from build123d import *

# Parameters (mm, degrees)
SKETCH1_W                                        = 55
SKETCH1_H                                        = 30
BOSS_EXTRUDE1_DEPTH                              = 10
SKETCH3_W                                        = 16.992180867
SKETCH3_H                                        = 11.731003527
SKETCH3_W_2                                      = 16.707792902
SKETCH3_W_3                                      = 9.029317866
SKETCH3_H_2                                      = 11.700356954
CUT_EXTRUDE1_DEPTH                               = 33.882366095
CBORE_FOR_M2_HEX_HEAD_MACHINE_SCREW2_D           = 2.4
CBORE_FOR_M2_HEX_HEAD_MACHINE_SCREW2_CBORE_D     = 6.38
CBORE_FOR_M2_HEX_HEAD_MACHINE_SCREW2_CBORE_DEPTH = 1.6
M3X0_5_TAPPED_HOLE3_D                            = 2.5
M3X0_5_TAPPED_HOLE3_DEPTH                        = 3
M3X0_5_TAPPED_HOLE3_TIP                          = 0.751075774


with BuildPart() as part:
    # Sketch1 → Boss-Extrude1 (new body)
    with BuildSketch(Plane.XY):
        Rectangle(SKETCH1_W, SKETCH1_H)
    extrude(amount=BOSS_EXTRUDE1_DEPTH)

    # Sketch3 → Cut-Extrude1 (cut, through all)
    with BuildSketch(Plane.XY.offset(10)):
        with Locations((-16.316759452, 0.350583033)):
            Rectangle(SKETCH3_W, SKETCH3_H)
        with Locations((4.016979996, 0.421680025)):
            Rectangle(SKETCH3_W_2, SKETCH3_H)
        with Locations((20.938063871, 0.193065764)):
            Rectangle(SKETCH3_W_3, SKETCH3_H_2)
    extrude(amount=-CUT_EXTRUDE1_DEPTH, mode=Mode.SUBTRACT)

    # CBORE for M2 Hex Head Machine Screw2 (through all)
    with Locations(Plane.XY.offset(10)):
        with Locations((-22.5, -10.5), (22.5, -10.5)):
            CounterBoreHole(CBORE_FOR_M2_HEX_HEAD_MACHINE_SCREW2_D / 2, CBORE_FOR_M2_HEX_HEAD_MACHINE_SCREW2_CBORE_D / 2, CBORE_FOR_M2_HEX_HEAD_MACHINE_SCREW2_CBORE_DEPTH)

    # M3x0.5 Tapped Hole3
    with Locations(Plane(origin=(0, 15, 0), x_dir=(1, 0, 0), z_dir=(0, 1, 0))):
        with Locations((-20.191545465, -5), (20.191545465, -5)):
            Hole(M3X0_5_TAPPED_HOLE3_D / 2, depth=M3X0_5_TAPPED_HOLE3_DEPTH)
            with Locations((0, 0, -(M3X0_5_TAPPED_HOLE3_DEPTH + M3X0_5_TAPPED_HOLE3_TIP / 2))):  # 118° drill point
                Cone(0, M3X0_5_TAPPED_HOLE3_D / 2, M3X0_5_TAPPED_HOLE3_TIP, mode=Mode.SUBTRACT)

    # Sketch12 → M3x0.5 Tapped Hole2 (revolve, cut)
    with BuildSketch(Plane(origin=(-27.5, -10, 5), x_dir=(0, 0, 1), z_dir=(0, 1, 0))):
        Polygon((0, 0), (0, 3.751075774), (1.25, 3), (1.25, 0), align=None)
    m3x0_5_tapped_hole2 = revolve(axis=Axis((-33.85, -10, 5), (1, 0, 0)), mode=Mode.SUBTRACT)

    # Sketch16 → M3x0.5 Tapped Hole1 (revolve, cut)
    with BuildSketch(Plane(origin=(27.5, -10, 5), x_dir=(0, 0, -1), z_dir=(0, 1, 0))):
        Polygon((0, 0), (0, 3.751075774), (1.25, 3), (1.25, 0), align=None)
    m3x0_5_tapped_hole1 = revolve(axis=Axis((33.85, -10, 5), (-1, 0, 0)), mode=Mode.SUBTRACT)

    # Mirror1: M3x0.5 Tapped Hole1 across plane
    add(m3x0_5_tapped_hole1.mirror(Plane.ZX), mode=Mode.SUBTRACT)

    # Mirror2: M3x0.5 Tapped Hole2 across plane
    add(m3x0_5_tapped_hole2.mirror(Plane.ZX), mode=Mode.SUBTRACT)


solid = part.part
Work out the finished part from the listing and answer in its coordinate system (mm). A direction names the side the tool comes from. Give positions to 0.01 mm unless a question says otherwise; leave off trailing zeros. Loops run counter-clockwise (first coordinate to the right, second up) from the corner with the lowest first, then second, coordinate; pieces in that order, holes last. Notation, with made-up numbers: (-38, -35) -> (-15, -35) arc R20 cw to (-15, -9) -> close; hole circle Ø5 at (11, 71.5). An arc over 180 degrees is marked (long way). Use a Markdown table: item, result. Add a question column.
1) The part is cut by section D-D, the plane z = 2.25. Determine the outline of the cut face in (x, y), plus the area to 3 significant figures.
2) The part is cut by section C-C, the plane x = -11.5. Determine the outline of the cut face in (y, z), plus the area to 3 significant figures.
3) Each of these flat-tipped pins is pushed along its axis until it touches: P1, Ø3, axis at x = 21.5, y = -11.5, coming from the +Z side; P2, Ø2, axis at y = -10, z = 5, coming from the +X side; P3, Ø2, axis at x = 20.19, z = 5, coming from the +Y side. Where does it stop, or does it pass through?
4) The part is cut by section B-B, the plane x = -22.5. Determine the outline of the cut face in (y, z).
5) Consider line 1 along X through (y, z) = (2.5, 5.5); line 2 along Y through (x, z) = (25.65, 5); line 3 along Y through (x, z) = (22.5, 9.1). Determine where each line is inside the solid, lowest interval first.
6) For a pull along X with two mould halves and no side action, classify faces 4 (the flat face through (27.5, 0, 5)), 5 (the flat face through (24, -10, 8.4)), 6 (the cylindrical face through (26.02, -11.24, 5.16)), 7 (the flat face through (-27.5, 0, 5)) as +X half, -X half, draft (parallel to the pull), parting line (faces both ways), or undercut.
7) The part is cut by section A-A, the plane z = 9.25. Determine the outline of the cut face in (x, y), plus the area to 3 significant figures.
8) Which of the six approach directions +Z, -Z, +X, -X, +Y, -Y give full straight-line access (tool end or side, diameter ignored) to faces 1 (the flat face through (0, -15, 5)), 2 (the flat face through (25.453, 0, 5)), 3 (the cylindrical face through (-21.346, 13.479, 5.479))?
Reported:
| question | item | result |
|---|---|---|
| 1 | outline | (-27.5, -15) -> (27.5, -15) -> (27.5, 15) -> (-27.5, 15) -> close; hole (-24.81, -5.51) -> (-7.82, -5.51) -> (-7.82, 6.22) -> (-24.81, 6.22) -> close; hole circle Ø2.4 at (-22.5, -10.5); hole (-4.34, -5.44) -> (12.37, -5.44) -> (12.37, 6.29) -> (-4.34, 6.29) -> close; hole (16.42, -5.66) -> (25.45, -5.66) -> (25.45, 6.04) -> (16.42, 6.04) -> close; hole circle Ø2.4 at (22.5, -10.5) |
| 1 | area | 1,140 mm^2 |
| 2 | outline | (-15, 0) -> (-5.51, 0) -> (-5.51, 10) -> (-15, 10) -> close; (6.22, 0) -> (15, 0) -> (15, 10) -> (6.22, 10) -> close |
| 2 | area | 183 mm^2 |
| 3 | P1 | stops at z = 8.4 |
| 3 | P2 | stops at x = 24.35 |
| 3 | P3 | stops at y = 11.85 |
| 4 | outline | (-15, 0) -> (-11.7, 0) -> (-11.7, 8.4) -> (-13.69, 8.4) -> (-13.69, 10) -> (-15, 10) -> close; (-9.3, 0) -> (-5.51, 0) -> (-5.51, 10) -> (-7.31, 10) -> (-7.31, 8.4) -> (-9.3, 8.4) -> close; (6.22, 0) -> (15, 0) -> (15, 10) -> (6.22, 10) -> close |
| 5 | line 1 | x = -27.5 to -24.81, -7.82 to -4.34, 12.37 to 16.42, 25.45 to 27.5 |
| 5 | line 2 | y = -15 to -11.25, -8.75 to 8.75, 11.25 to 15 |
| 5 | line 3 | y = -15 to -13.69, -7.31 to -5.66, 6.04 to 15 |
| 6 | face 4 | +X half |
| 6 | face 5 | undercut |
| 6 | face 6 | draft |
| 6 | face 7 | -X half |
| 7 | outline | (-27.5, -15) -> (27.5, -15) -> (27.5, 15) -> (-27.5, 15) -> close; hole circle Ø6.38 at (-22.5, -10.5); hole (-24.81, -5.51) -> (-7.82, -5.51) -> (-7.82, 6.22) -> (-24.81, 6.22) -> close; hole (-4.34, -5.44) -> (12.37, -5.44) -> (12.37, 6.29) -> (-4.34, 6.29) -> close; hole (16.42, -5.66) -> (25.45, -5.66) -> (25.45, 6.04) -> (16.42, 6.04) -> close; hole circle Ø6.38 at (22.5, -10.5) |
| 7 | area | 1,090 mm^2 |
| 8 | face 1 | +Z, -Z, +X, -X, -Y |
| 8 | face 2 | +Z, -Z |
| 8 | face 3 | +Y |
